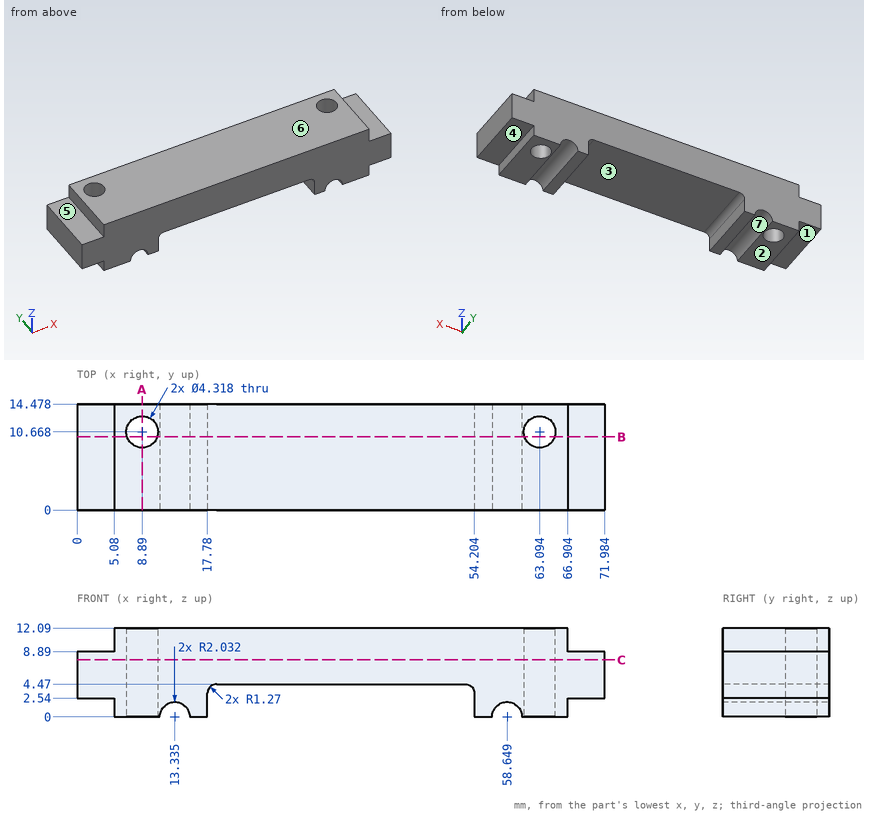
Could you check a few things on this drawing? It's one solid part, dimensions in mm from its lowest x, y, z. A direction names the side the tool comes from. Give positions to 0.01 mm unless a question says otherwise; leave off trailing zeros. Order: outer loops, then holes, each group sorted by start corner. A loop starts at its lowest first (then second) coordinate and runs counter-clockwise, first axis right, second up. Notation, with made-up numbers: (6.5, -17.75) -> (52.5, -17.75) arc R12 ccw to (52.5, -4.75) -> close; hole circle Ø5 at (39, -35). An arc over 180 degrees is marked (long way). Use CSV: the item, a comma, the result in double quotes. Start each with the question number.
Item 1: I'm going to push flat-ended pins straight in: P1, Ø1.5, axis at y = 10, z = 11, coming from the +X side; P2, Ø1, axis at y = 7, z = 10, coming from the -X side; P3, Ø3, axis at y = 13, z = 9, coming from the +X side; P4, Ø2.5, axis at x = 69.5, y = 9.5, coming from the +Z side. Where does each tip first touch, or does it pass through?
Item 2: If I drill on probe 1 along Y at (x, z) = (9, 4.75) (1 decimal); probe 2 along Z at (x, y) = (50, 10.25); probe 3 along X at (y, z) = (11.5, 8.5) (1 decimal), over which ranges is the centre line in solid material (lowest first)? Write a range as [from, to].
Item 3: Thinking about a two-plate mould opening in X: for the marked faces 6 and 7, which applies, pulls with the +X half, pulls with the -X half, needs draft (parallel to the pull), parting line crosses it, or undercut?
Item 4: On a 3-axis mill with a long thin cutter (end or side, diameter ignored), from which of +Z, -Z, +X, -X, +Y, -Y can I reach the whole of each face in a straight line? I mean the marked faces 1, 2, 3, 4 and 5. Say none if no direction works.
Item 5: Suppose I cut it at B-B (y = 10). Give the number of separate pieces and of enclosed holes in the cut face.
Item 6: Suppose I cut it at A-A (x = 8.89). List the corners of the cut face in (y, z) for me.
Item 7: Suppose I cut it at C-C (z = 7.75). List the corners of the cut face in (x, y) for me, and give its area (3 significant figures).
Answer block:
1,P1,"stops at x = 66.9"
1,P2,"stops at x = 5.08"
1,P3,"stops at x = 71.98"
1,P4,"stops at z = 8.89"
2,probe 1,"y = [0, 8.5], [12.8, 14.5]"
2,probe 2,"z = [4.47, 12.09]"
2,probe 3,"x = [0, 6.9], [10.9, 61.1], [65.1, 72]"
3,face 6,"needs draft"
3,face 7,"undercut"
4,face 1,"-Z, -X, +Y, -Y"
4,face 2,"-Z, +X, -X, +Y, -Y"
4,face 3,"-Z, +Y, -Y"
4,face 4,"-Z, +X, +Y, -Y"
4,face 5,"+Z, -X, +Y, -Y"
5,separate pieces,"3"
5,enclosed holes,"0"
6,outline,"(0, 0) -> (8.51, 0) -> (8.51, 12.09) -> (0, 12.09) -> close; (12.83, 0) -> (14.48, 0) -> (14.48, 12.09) -> (12.83, 12.09) -> close"
7,outline,"(0, 0) -> (71.98, 0) -> (71.98, 14.48) -> (0, 14.48) -> close; hole circle Ø4.32 at (8.89, 10.67); hole circle Ø4.32 at (63.09, 10.67)"
7,area,"1,010 mm^2"
